CAD build for the part. Positions are in the model's coordinates, mm. Face numbers are marked on the shaded views. A direction names the side the tool comes from. Coordinates: 2 decimals unless noted, no trailing zeros. Order: outer loops, then holes, each group sorted by start corner. A loop starts at its lowest first (then second) coordinate and runs counter-clockwise, first axis right, second up. Notation, with made-up numbers: M -22.5,11 L -11.5,11 A24 cw -11.5,41 Z; hole C -25,24.25 d10. An arc over 180 degrees is marked long. Write item = value, one per line. Start each with the question number.
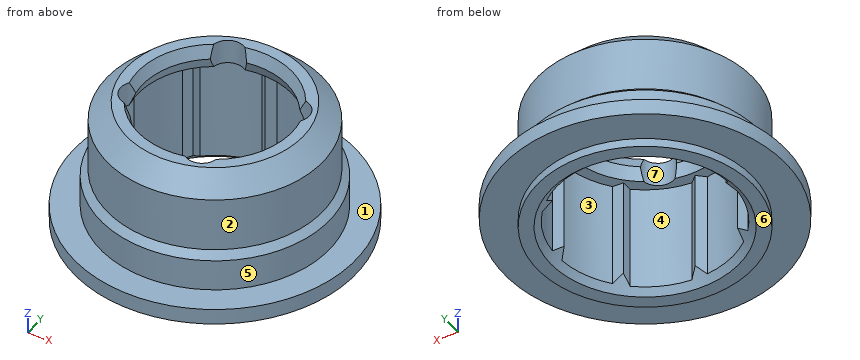
```python
from build123d import *

# Parameters (mm, degrees)
PAD_DEPTH             = 4.6
POLARPATTERN004_COUNT = 8
SKETCH010_R           = 0.65
POCKET001_DEPTH       = 40.002163
POLARPATTERN005_COUNT = 4


with BuildPart() as part:
    # Sketch007 → Revolution005 (revolve)
    with BuildSketch(Plane.XZ):
        Polygon((-3.6, 4.6), (-3.6, 3.5), (-3.6, 2.5), (-3.6, 1), (-3.6, 0), (-4.4, 0), (-4.4, 0.35), (-5.75, 0.35), (-5.75, 1), (-4.675, 1), (-4.675, 2.3), (-4.4, 2.575), (-4.4, 4.8), (-3.6, 5.6), (-3.15, 5.6), (-2.95, 5.1), (-3.15, 4.6), align=None)
    revolve(axis=Axis((0, 0, 0), (0, 0, 1)))

    # Sketch008 → Pad (new body)
    with BuildSketch(Plane.XY):
        with BuildLine():
            ThreePointArc((-3.586301, 0.313761), (-3.6, 0), (-3.586301, -0.313761))
            Line((-3.3, 0), (-3.586301, -0.313761))
            Line((-3.586301, 0.313761), (-3.3, 0))
        make_face()
    pad = extrude(amount=PAD_DEPTH)

    # PolarPattern004: Pad ×8 about axis
    polarpattern004_axis = Axis((0, 0, 0), (0, 0, 1))
    for i in range(1, POLARPATTERN004_COUNT):
        add(pad.rotate(polarpattern004_axis, i * 360 / POLARPATTERN004_COUNT))

    # Sketch009 → Groove (revolve, cut)
    with BuildSketch(Plane.XZ):
        Polygon((-3.85, 0), (0, 3.85), (0, 0), align=None)
    revolve(axis=Axis((0, 0, 0), (0, 0, 1)), mode=Mode.SUBTRACT)

    # Sketch010 → Pocket001 (cut, through all)
    with BuildSketch(Plane.XY):
        with Locations((2.540669, 1.052379)):
            Circle(SKETCH010_R)
    pocket001 = extrude(amount=POCKET001_DEPTH, mode=Mode.SUBTRACT)

    # PolarPattern005: Pocket001 ×4 about axis
    polarpattern005_axis = Axis((0, 0, 0), (0, 0, 1))
    for i in range(1, POLARPATTERN005_COUNT):
        add(pocket001.rotate(polarpattern005_axis, i * 360 / POLARPATTERN005_COUNT), mode=Mode.SUBTRACT)


solid = part.part
```
1. Flat gauge pin, fed straight in: pin 1 (1.5 mm diameter, centred on y = -4, z = 4, fed in from -X). Where does the tip first touch, or does it go through?
2. 3-axis set-ups, long thin cutter, end or side, ignore diameter. For the marked faces 4, 5, 6 and 7: which of +Z, -Z, +X, -X, +Y, -Y reach the whole face in a straight line?
3. Probe L1, parallel to Z at x = -0.5, y = 3.5; L2, parallel to X at y = -3.25, z = 1.5; L3, parallel to Y at x = -3, z = 2.4. List the from-to ranges inside material, lowest first.
4. Slice it at B-B (z = 1.4). Write the cut outline in (x, y) (3 decimals), plus the area to 3 significant figures.
5. Slice it at A-A (z = 3.35). Write the cut outline in (x, y).
6. Mould opens along X. For the marked faces 1, 2 and 3 say: released by +X, released by -X, zero draft, split by the parting line, or undercut.
7. Slice it at C-C (z = 5.25). Write the cut outline in (x, y), plus the area to 3 significant figures.
Calculated:
q1.pin_1 = -2.97
q2.face_4 = -Z
q2.face_5 = +Z
q2.face_6 = -Z, +X, -X, +Y, -Y
q2.face_7 = +Z, -Z
q3.L1 = 4.6 to 5.6
q3.L2 = -3.36 to -1.55, 1.55 to 3.36
q3.L3 = -3.45 to -1.99, 1.99 to 3.45
q4.outline = C 0,0 d9.35; hole M -3.586,-0.314 A3.6 ccw -2.758,-2.314 L -2.333,-2.333 L -2.314,-2.758 A3.6 ccw -0.314,-3.586 L 0,-3.3 L 0.314,-3.586 A3.6 ccw 2.314,-2.758 L 2.333,-2.333 L 2.758,-2.314 A3.6 ccw 3.586,-0.314 L 3.3,0 L 3.586,0.314 A3.6 ccw 2.758,2.314 L 2.333,2.333 L 2.314,2.758 A3.6 ccw 0.314,3.586 L 0,3.3 L -0.314,3.586 A3.6 ccw -2.314,2.758 L -2.333,2.333 L -2.758,2.314 A3.6 ccw -3.586,0.314 L -3.3,0 Z
q4.area = 28.7 mm²
q5.outline = C 0,0 d8.8; hole M -3.59,-0.31 A3.6 ccw -2.76,-2.31 L -2.33,-2.33 L -2.31,-2.76 A3.6 ccw -0.31,-3.59 L 0,-3.3 L 0.31,-3.59 A3.6 ccw 2.31,-2.76 L 2.33,-2.33 L 2.76,-2.31 A3.6 ccw 3.59,-0.31 L 3.3,0 L 3.59,0.31 A3.6 ccw 2.76,2.31 L 2.33,2.33 L 2.31,2.76 A3.6 ccw 0.31,3.59 L 0,3.3 L -0.31,3.59 A3.6 ccw -2.31,2.76 L -2.33,2.33 L -2.76,2.31 A3.6 ccw -3.59,0.31 L -3.3,0 Z
q6.face_1 = zero draft
q6.face_2 = split by the parting line
q6.face_3 = undercut
q7.outline = C 0,0 d7.9; hole M -2.96,-0.55 A0.65 ccw -2.48,-1.7 A3.01 ccw 0.55,-2.96 A0.65 ccw 1.7,-2.48 A3.01 ccw 2.96,0.55 A0.65 ccw 2.48,1.7 A3.01 ccw -0.55,2.96 A0.65 ccw -1.7,2.48 A3.01 ccw Z
q7.area = 19.1 mm²
